from build123d import *

# Parameters (mm, degrees)
CORTAR_EXTRUIR1_DEPTH = 4
CHAFL_N1_SIZE         = 0.5


with BuildPart() as part:
    # Croquis1 → Revolución1 (revolve)
    with BuildSketch(Plane(origin=(0, 0, 0), x_dir=(-1, 0, 0), z_dir=(0, 1, 0)), mode=Mode.PRIVATE) as revoluci_n1_sk:
        Polygon((-19.1, 3), (19.1, 3), (19.1, 2.85), (19.9, 2.85), (19.9, 3), (24.1, 3), (24.1, 0), (-24.1, 0), (-24.1, 3), (-19.9, 3), (-19.9, 2.85), (-19.1, 2.85), align=None)
    revolve(revoluci_n1_sk.sketch.rotate(Axis((24.1, 0, 0), (-1, 0, 0)), 180), axis=Axis((24.1, 0, 0), (-1, 0, 0)))

    # Croquis2 → Cortar-Extruir1 (cut, symmetric)
    with BuildSketch(Plane.YZ):
        with BuildLine():
            Line((1.658312395, 2.5), (-1.658312395, 2.5))
            ThreePointArc((-1.658312395, 2.5), (0, 3), (1.658312395, 2.5))
        make_face()
    extrude(amount=CORTAR_EXTRUIR1_DEPTH, both=True, mode=Mode.SUBTRACT)

    # Chaflán1
    chafl_n1_edges = [part.edges().sort_by_distance(p)[0] for p in [
        (24.1, 0, 3),
        (-24.1, 0, 3),
    ]]
    chamfer(chafl_n1_edges, length=CHAFL_N1_SIZE)


solid = part.part
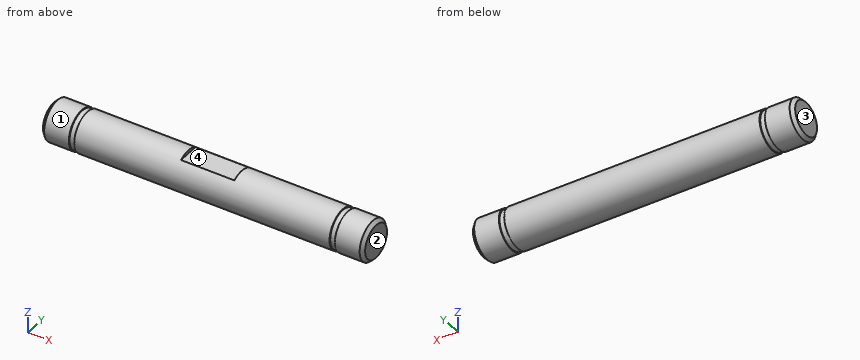
Verification items for the finished model (mm, model axes). Face numbers are marked on the shaded views. Coordinates: 2 decimals unless noted, no trailing zeros. Order: outer loops, then holes, each group sorted by start corner. A loop starts at its lowest first (then second) coordinate and runs counter-clockwise, first axis right, second up. Notation, with made-up numbers: M -25,56.5 L -1,56.5 A29 ccw -1,77.5 Z; hole C -18,72.25 d3. An arc over 180 degrees is marked long. One line per item, written item: value. Start each with the question number.
Item 1: Thickness scan on probe 1 along X at (y, z) = (-0.9, 2.75); probe 2 along Y at (x, z) = (-1, -2.5); probe 3 along Z at (x, y) = (-10, -0.2). Record the ranges inside material, lowest first.
Item 2: Sectioned sample at B-B on x = 6.5. Record the cut outline in (y, z).
Item 3: Mould release check, pull along X, two halves, no side actions. Record for the marked faces 1, 2, 3 and 4: pulls with the +X half, pulls with the -X half, needs draft (parallel to the pull), parting line crosses it, or undercut.
Item 4: Sectioned sample at A-A on y = 0. Record the cut outline in (x, z).
Item 5: Depth check by flat-ended pin: P1, Ø1, axis at x = 9, y = 1.5, coming from the -Z side; P2, Ø1.5, axis at x = 7.5, z = -2.5, coming from the +Y side; P3, Ø2, axis at x = -3.5, y = 1.5, coming from the +Z side. Enter the tip coordinate at first touch or a pass-through.
Calculated:
1. probe 1: -23.71 to -19.9, -19.1 to -4, 4 to 19.1, 19.9 to 23.71
1. probe 2: -1.66 to 1.66
1. probe 3: -2.99 to 2.99
2. outline: C 0,0 d6
3. face 1: needs draft
3. face 2: pulls with the +X half
3. face 3: pulls with the -X half
3. face 4: undercut
4. outline: M -24.1,-2.5 L -23.6,-3 L -19.9,-3 L -19.9,-2.85 L -19.1,-2.85 L -19.1,-3 L 19.1,-3 L 19.1,-2.85 L 19.9,-2.85 L 19.9,-3 L 23.6,-3 L 24.1,-2.5 L 24.1,2.5 L 23.6,3 L 19.9,3 L 19.9,2.85 L 19.1,2.85 L 19.1,3 L 4,3 L 4,2.5 L -4,2.5 L -4,3 L -19.1,3 L -19.1,2.85 L -19.9,2.85 L -19.9,3 L -23.6,3 L -24.1,2.5 Z
5. P1: z = -2.83
5. P2: y = 2.44
5. P3: z = 2.93
